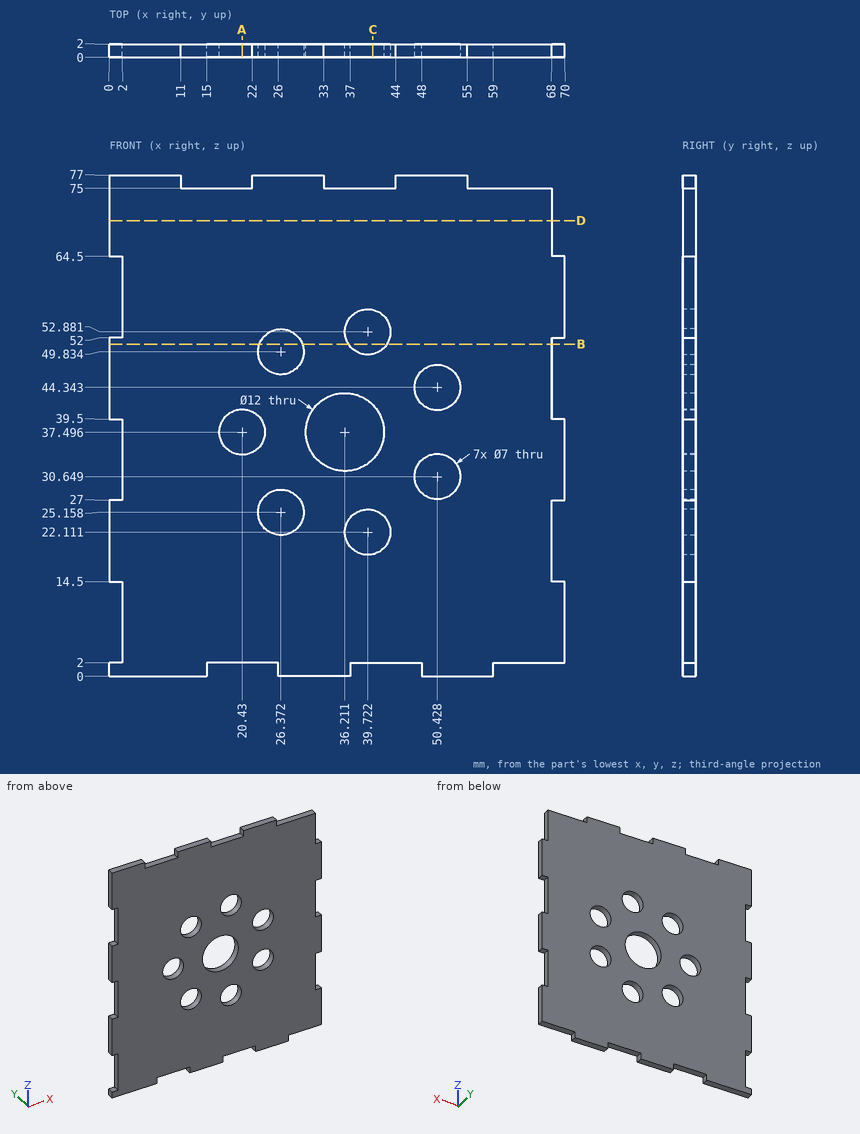
Can you work these out from the drawing? Everything is in mm from the part's minimum corner. Coordinates: 2 decimals unless noted, no trailing zeros. Loops run counter-clockwise (first coordinate to the right, second up) from the corner with the lowest first, then second, coordinate; pieces in that order, holes last. Notation, with made-up numbers: (29, 55) - (74, 55) arc R17 cw to (74, 67) - close; hole circle Ø6 at (-35.75, 62.25). An arc over 180 degrees is marked (long way). Use a Markdown table: item, result.
Item 1: I want a section at A-A on x = 20.43. Please give me the cut outline in (y, z) (1 decimal), and give its area (3 significant figures).
Numbers:
| item | result |
|---|---|
| outline | (0, 2) - (2, 2) - (2, 34) - (0, 34) - close; (0, 41) - (2, 41) - (2, 75) - (0, 75) - close |
| area | 132 mm2 |
Item 2: I want a section at D-D on z = 70. Please give me the cut outline in (x, y), and give its area (3 significant figures).
Numbers:
| item | result |
|---|---|
| outline | (0, 0) - (68, 0) - (68, 2) - (0, 2) - close |
| area | 136 mm2 |
Item 3: If I drill on probe 1 along X at (y, z) = (0.65, 22) (1 decimal); probe 2 along Z at (x, y) = (47.5, 1.65) (1 decimal); probe 3 along X at (y, z) = (1.2, 24) (1 decimal), over which ranges is the centre line in solid material (lowest first)? Write a range as from..to.
Numbers:
| item | result |
|---|---|
| probe 1 | x = 0..24.9, 27.9..36.2, 43.2..68 |
| probe 2 | z = 2..28.7, 32.6..42.4, 46.3..77 |
| probe 3 | x = 0..23.1, 29.7..36.8, 42.7..68 |
Item 4: I want a section at C-C on x = 40.5. Please give me the cut outline in (y, z).
Numbers:
| item | result |
|---|---|
| outline | (0, 2) - (2, 2) - (2, 18.7) - (0, 18.7) - close; (0, 25.52) - (2, 25.52) - (2, 33.3) - (0, 33.3) - close; (0, 41.69) - (2, 41.69) - (2, 49.47) - (0, 49.47) - close; (0, 56.29) - (2, 56.29) - (2, 75) - (0, 75) - close |
Item 5: I want a section at B-B on z = 51. Please give me the cut outline in (x, y) (1 decimal), and give its area (3 significant figures).
Numbers:
| item | result |
|---|---|
| outline | (0, 0) - (23.1, 0) - (23.1, 2) - (0, 2) - close; (29.7, 0) - (36.8, 0) - (36.8, 2) - (29.7, 2) - close; (42.7, 0) - (68, 0) - (68, 2) - (42.7, 2) - close |
| area | 111 mm2 |
Item 6: Will these pins go through, and if not, where does the flat tip stop? pin 1 (0.6 mm diameter, centred on y = 1.5, z = 20, fed in from +X); pin 2 (0.6 mm diameter, centred on x = 66, y = 1, fed in from -Z).
Numbers:
| item | result |
|---|---|
| pin 1 | stops at x = 68 |
| pin 2 | stops at z = 2 |
